```python
from build123d import *

# Parameters (mm, degrees)
F0_W     = 88.9
F0_H     = 69.85
F1_DEPTH = 869.95
F2_W     = 25.4
F2_H     = 12.7
F3_DEPTH = 12.7
F4_W     = 63.5
F4_H     = 12.7
F5_DEPTH = 88.9
F6_W     = 88.9
F6_H     = 12.7
F7_DEPTH = 88.9


with BuildPart() as f1:
    # F0 (on Front) → F1 (new body)
    with BuildSketch(Plane.XZ):
        with Locations((44.45, 23.882015)):
            Rectangle(F0_W, F0_H)
    extrude(amount=F1_DEPTH)

    # F2 (on face) → F3 (cut)
    with BuildSketch(Plane.YZ.offset(88.9)):
        with Locations((-857.25, 23.882015)):
            Rectangle(F2_W, F2_H)
    extrude(amount=-F3_DEPTH, mode=Mode.SUBTRACT)

    # F4 (on face) → F5 (cut, through all)
    with BuildSketch(Plane.YZ.offset(88.9)):
        with Locations((-812.8, 23.882015)):
            Rectangle(F4_W, F4_H)
    extrude(amount=-F5_DEPTH, mode=Mode.SUBTRACT)

    # F6 (on face) → F7 (cut, through all)
    with BuildSketch(Plane.YZ.offset(88.9)):
        with Locations((-247.65, 23.882015)):
            Rectangle(F6_W, F6_H)
    extrude(amount=-F7_DEPTH, mode=Mode.SUBTRACT)


solid = f1.part
```
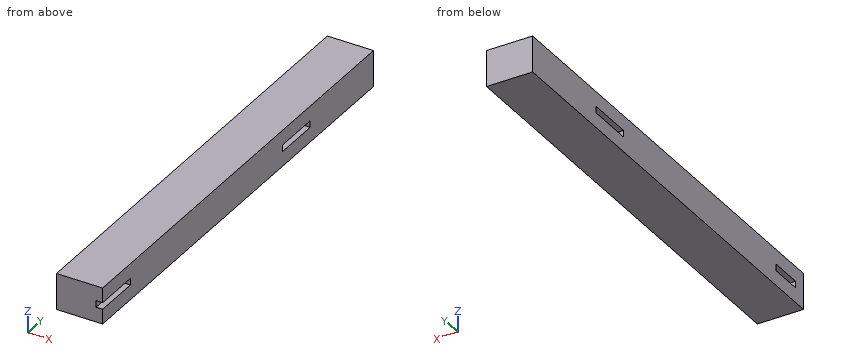
Part model, mm, in its own coordinate system. Round coordinates to 2 decimals unless told otherwise and drop trailing zeros. Loops run counter-clockwise (first coordinate to the right, second up) from the corner with the lowest first, then second, coordinate; pieces in that order, holes last. Notation, with made-up numbers: (-19, 50.25) -> (35, 50.25) arc R23 cw to (35, 64.25) -> close; hole circle Ø5 at (35.25, -35). An arc over 180 degrees is marked (long way). Use a Markdown table: item, result.
1) Drop a flat-ended pin along its axis: pin 1 Ø10 at (x, z) = (36.5, 24) entering from +Y. Give the stop position or say it passes through.
The answers:
| item | result |
|---|---|
| pin 1 | stops at y = 0 |
2) Cut at A-A, the plane y = -213. List the corners of the cut face in (x, z).
The answers:
| item | result |
|---|---|
| outline | (0, -11.04) -> (88.9, -11.04) -> (88.9, 17.53) -> (0, 17.53) -> close; (0, 30.23) -> (88.9, 30.23) -> (88.9, 58.81) -> (0, 58.81) -> close |
3) Probe line 1 (Y direction, x = 11, z = 19.5); line 2 (Z direction, x = 82.5, y = -215). List the from-to ranges inside material, lowest first. Write a range as [from, to].
The answers:
| item | result |
|---|---|
| line 1 | y = [-869.95, -844.55], [-781.05, -292.1], [-203.2, 0] |
| line 2 | z = [-11.04, 17.53], [30.23, 58.81] |
4) Cut at B-B, the plane x = 65. List the corners of the cut face in (y, z), and give its area (3 significant figures).
The answers:
| item | result |
|---|---|
| outline | (-869.95, -11.04) -> (0, -11.04) -> (0, 58.81) -> (-869.95, 58.81) -> close; hole (-844.55, 17.53) -> (-781.05, 17.53) -> (-781.05, 30.23) -> (-844.55, 30.23) -> close; hole (-292.1, 17.53) -> (-203.2, 17.53) -> (-203.2, 30.23) -> (-292.1, 30.23) -> close |
| area | 58,800 mm2 |
